Geometry check sheet. Reference: the model listing, model coordinates, mm. Coordinates: 2 decimals unless noted, no trailing zeros. Loops run counter-clockwise (first coordinate to the right, second up) from the corner with the lowest first, then second, coordinate; pieces in that order, holes last. Notation, with made-up numbers: (81.5, -31) - (130.5, -31) arc R26 ccw to (130.5, -15) - close; hole circle Ø4 at (25, 75.25). An arc over 180 degrees is marked (long way). One line per item, written item: value.
from build123d import *

# Parameters (mm, degrees)
F0_W     = 110
F0_H     = 100
F0_R     = 2
F0_R_2   = 5
F1_DEPTH = 10


with BuildPart() as f1:
    # F0 (on Front) → F1 (new body)
    with BuildSketch(Plane.XZ):
        Rectangle(F0_W, F0_H)
        with Locations((-50, -30)):
            Circle(F0_R, mode=Mode.SUBTRACT)
        with Locations((-25, -45)):
            Circle(F0_R, mode=Mode.SUBTRACT)
        with Locations((35, -45)):
            Circle(F0_R, mode=Mode.SUBTRACT)
        with Locations((-30, 0)):
            Circle(F0_R_2, mode=Mode.SUBTRACT)
        with Locations((-50, 30)):
            Circle(F0_R, mode=Mode.SUBTRACT)
    extrude(amount=F1_DEPTH)


solid = f1.part
(1) Release check for a two-part mould opening along Z. For faces 1 (the face through (55, -5, -1)), 2 (the face through (-50, -5, 28)), 3 (the face through (-1, -5, -50)) record: pulls with the +Z half, pulls with the -Z half, needs draft (parallel to the pull), parting line crosses it, or undercut.
Reply:
face 1: needs draft
face 2: undercut
face 3: pulls with the -Z half
(2) Material ranges on probe 1 along Z at (x, y) = (35, -6); probe 2 along Z at (x, y) = (-24.5, -0.75); probe 3 along X at (y, z) = (-0.75, -29), recorded low to high. Write a range as from..to.
Reply:
probe 1: -50..-47, -43..50
probe 2: -50..-46.94, -43.06..50
probe 3: -55..-51.73, -48.27..55
(3) Go/stop test with a flat-tipped pin: pin 1 Ø6.5 at (x, z) = (-50, -30) entering from +Y. Record where the tip stops, or that it passes through.
Reply:
pin 1: y = 0
(4) Cross-section at C-C on x = 35. Record the cut outline in (y, z).
Reply:
outline: (-10, -50) - (0, -50) - (0, -47) - (-10, -47) - close; (-10, -43) - (0, -43) - (0, 50) - (-10, 50) - close
(5) Cross-section at D-D on z = -30. Record the cut outline in (x, y).
Reply:
outline: (-55, -10) - (-52, -10) - (-52, 0) - (-55, 0) - close; (-48, -10) - (55, -10) - (55, 0) - (-48, 0) - close
(6) Cross-section at A-A on x = -50. Record the cut outline in (y, z).
Reply:
outline: (-10, -50) - (0, -50) - (0, -32) - (-10, -32) - close; (-10, -28) - (0, -28) - (0, 28) - (-10, 28) - close; (-10, 32) - (0, 32) - (0, 50) - (-10, 50) - close
(7) Cross-section at B-B on z = -45. Record the cut outline in (x, y), and give its area (3 significant figures).
Reply:
outline: (-55, -10) - (-27, -10) - (-27, 0) - (-55, 0) - close; (-23, -10) - (33, -10) - (33, 0) - (-23, 0) - close; (37, -10) - (55, -10) - (55, 0) - (37, 0) - close
area: 1,020 mm2
